Read the model definition and answer for the solid it produces. Units are mm, in the model's axes. Give positions to 0.01 mm unless a question says otherwise; leave off trailing zeros. Write each loop counter-clockwise with the first axis right and the second up, starting at its lowest first coordinate (ties: lowest second). Pieces come first, ordered by that corner, then holes. Notation, with made-up numbers: (39, 79.25) - (89, 79.25) arc R8 cw to (89, 91.25) - close; hole circle Ø3 at (28.25, 58.5). An arc over 180 degrees is marked (long way). Answer as CSV lines item,"result".
Autodesk Fusion 360 part; units mm, degrees
sketch "Sketch1" plane through (0, 0, 0) normal (0, 0, 1) x (1, 0, 0)
  line L0 (-100, 50) -> (300, 50)
  line L1 (300, 50) -> (300, -350)
  line L2 (300, -350) -> (-100, -350)
  line L3 (-100, -350) -> (-100, 50)
  dimension "d1" = 400
  dimension "d2" = 400
extrude "Extrude1" add sketch "Sketch1" along normal blind 3
sketch "Sketch2" plane through (0, 0, 3) normal (0, 0, 1) x (-1, 0, 0)
  line L0 (100, 350) -> (-300, 350)
  line L1 (-300, 350) -> (-300, -50)
  line L2 (-300, -50) -> (100, -50)
  line L3 (100, -50) -> (100, 350)
  line L4 (-263.3486, -40) -> (-290, -13.1239)
  line L5 (-290, -13.1239) -> (-270.7994, 7.2868)
  line L6 (-270.7994, 7.2868) -> (-243.7577, -19.9951)
  line L7 (-243.7577, -19.9951) -> (-263.3486, -40)
  circle A0 centre (-263.3392, -37.3821) radius 1
  circle A1 centre (-287.4151, -13.0924) radius 1
  circle A2 centre (-246.3371, -20.0207) radius 1
  circle A3 centre (-270.413, 4.269) radius 1
  line L8 (-105, 220) -> (-270, 220)
  line L9 (-270, 220) -> (-270, 320)
  line L10 (-270, 320) -> (-105, 320)
  line L11 (-105, 320) -> (-105, 220)
  circle A4 centre (-130.5, 232.5) radius 2.5
  circle A5 centre (-130.5, 307.5) radius 2.5
  circle A6 centre (-182.5, 232.5) radius 2.5
  circle A7 centre (-182.5, 307.5) radius 2.5
  line L12 (-152.9998, 228.0039) -> (-160.7739, 228.0044) construction
  line L13 (-160.7739, 228.0044) -> (-160.7741, 225.0005) construction
  line L14 (-160.7741, 225.0005) -> (-153, 225) construction
  line L15 (-153, 225) -> (-152.9998, 228.0039) construction
  line L16 (-153, 315) -> (-168.7144, 314.9704) construction
  line L17 (-168.7144, 314.9704) -> (-168.6983, 306.4348) construction
  line L18 (-168.6983, 306.4348) -> (-152.9839, 306.4644) construction
  line L19 (-152.9839, 306.4644) -> (-153, 315) construction
  line L20 (-49.76, 127.68) -> (70, 127.68)
  circle A8 centre (67.5, 66.3) radius 1.25
  line L21 (70, 127.68) -> (70, 63.8)
  circle A9 centre (-47.26, 125.18) radius 1.25
  circle A10 centre (67.5, 125.18) radius 1.25
  line L22 (-49.76, 63.8) -> (-49.76, 127.68)
  circle A11 centre (-47.26, 66.3) radius 1.25
  line L23 (70, 63.8) -> (-49.76, 63.8)
  line L24 (70, -20) -> (6.9, -20)
  line L25 (70, 33.8) -> (70, -20)
  line L26 (6.9, -20) -> (6.9, 33.8)
  circle A12 centre (9.4, 31.3) radius 1.25
  circle A13 centre (9.4, -17.5) radius 1.25
  circle A14 centre (67.5, 31.3) radius 1.25
  circle A15 centre (67.5, -17.5) radius 1.25
  line L27 (6.9, 33.8) -> (70, 33.8)
  circle A16 centre (67.5, 197.68) radius 1.25
  line L28 (70, 157.68) -> (28.7, 157.68)
  circle A17 centre (67.5, 160.18) radius 1.25
  line L29 (70, 200.18) -> (70, 157.68)
  circle A18 centre (31.2, 197.68) radius 1.25
  line L30 (28.7, 200.18) -> (70, 200.18)
  line L31 (28.7, 157.68) -> (28.7, 200.18)
  circle A19 centre (31.2, 160.18) radius 1.25
  dimension "d5" = 2
  dimension "d6" = 2
  dimension "d7" = 2
  dimension "d8" = 2
  dimension "d9" = 34.2
  dimension "d10" = 24.3
  dimension "d11" = 34.2
  dimension "d12" = 24.3
  dimension "d13" = 37.85
  dimension "d14" = 28
  dimension "d15" = 1.85
  dimension "d16" = 1.85
  dimension "d17" = 1.85
  dimension "d18" = 1.825
  dimension "d19" = 1.825
  dimension "d20" = 100
  dimension "d21" = 165
  dimension "d22" = 5
  dimension "d23" = 5
  dimension "d24" = 5
  dimension "d25" = 5
  dimension "d26" = 52
  dimension "d27" = 75
  dimension "d28" = 52
  dimension "d29" = 75
  dimension "d30" = 25.5
  dimension "d31" = 25.5
  dimension "d32" = 12.5
  dimension "d33" = 10
  dimension "d34" = 10
  dimension "d35" = 87.5
  dimension "d36" = 12.5
  dimension "d37" = 5
  dimension "d38" = 48
  dimension "d39" = 5
  dimension "d40" = 48
  dimension "d190" = 10
  dimension "d42" = 2.5
  dimension "d43" = 2.5
  dimension "d44" = 2.5
  dimension "d45" = 2.5
  dimension "d46" = 2.5
  dimension "d47" = 2.5
  dimension "d48" = 2.5
  dimension "d49" = 2.5
  dimension "d50" = 2.5
  dimension "d51" = 2.5
  dimension "d52" = 2.5
  dimension "d53" = 114.76
  dimension "d54" = 58.88
  dimension "d55" = 58.88
  dimension "d56" = 2.5
  dimension "d57" = 114.76
  dimension "d186" = 10
  dimension "d59" = 2.5
  dimension "d60" = 2.5
  dimension "d61" = 2.5
  dimension "d62" = 2.5
  dimension "d63" = 2.5
  dimension "d64" = 2.5
  dimension "d65" = 2.5
  dimension "d66" = 2.5
  dimension "d67" = 2.5
  dimension "d68" = 2.5
  dimension "d69" = 2.5
  dimension "d70" = 58.1
  dimension "d71" = 48.8
  dimension "d72" = 48.8
  dimension "d188" = 10
  dimension "d74" = 2.5
  dimension "d75" = 2.5
  dimension "d76" = 2.5
  dimension "d77" = 2.5
  dimension "d78" = 2.5
  dimension "d79" = 2.5
  dimension "d80" = 2.5
  dimension "d81" = 2.5
  dimension "d82" = 2.5
  dimension "d83" = 2.5
  dimension "d84" = 2.5
  dimension "d85" = 37.5
  dimension "d86" = 36.3
  dimension "d87" = 36.3
  dimension "d90" = 30
  dimension "d91" = 58.1
  dimension "d92" = 30
  dimension "d93" = 30
  dimension "d94" = 30
  dimension "d95" = 30
  dimension "d96" = 30
  dimension "d97" = 12.5
  dimension "d98" = 87.5
  dimension "d99" = 10
  dimension "d100" = 10
  dimension "d101" = 30
  dimension "d102" = 30
sketch "Sketch3" plane through (0, 0, 3) normal (0, 0, 1) x (1, 0, 0)
  line L0 (-100, -350.18) -> (75, -350.18)
  line L1 (75, -350.18) -> (75, -230.18)
  line L2 (75, -230.18) -> (-100, -230.18)
  line L3 (-100, -230.18) -> (-100, -350.18)
  line L4 (-28.7, -200.18) -> (-70, -200.18)
  line L5 (105, -320) -> (105, -220)
  dimension "d103" = 30
  dimension "d104" = 30
  dimension "d105" = 120
  dimension "d106" = 175
extrude "Extrude2" cut sketch "Sketch3" against normal blind 5.5
extrude "Extrude3" cut sketch "Sketch2" against normal blind 5.5 contours A4 | A5 | A6 | A7 | A8 | A9 | A10 | A11 | A12 | A13 | A14 | A15 | A16 | A17 | A18 | A19
extrude "Extrude4" cut sketch "Sketch2" against normal blind 5.5 contours A0 | A1 | A2 | A3
sketch "Sketch4" plane through (0, 0, 3) normal (0, 0, 1) x (-1, 0, 0)
  circle A0 centre (-270.413, 4.269) radius 1
  circle A1 centre (-287.4151, -13.0924) radius 1
  circle A2 centre (-246.3371, -20.0207) radius 1
  circle A3 centre (-263.3392, -37.3821) radius 1
  circle A4 centre (9.4, 31.3) radius 1.25
  circle A5 centre (-47.26, 125.18) radius 1.25
  circle A6 centre (31.2, 160.18) radius 1.25
  circle A7 centre (-130.5, 232.5) radius 2.5
  circle A8 centre (-182.5, 307.5) radius 2.5
  circle A9 centre (67.5, 197.68) radius 1.25
  circle A10 centre (-47.26, 66.3) radius 1.25
  circle A11 centre (9.4, -17.5) radius 1.25
  circle A12 centre (67.5, 31.3) radius 1.25
  circle A13 centre (67.5, 125.18) radius 1.25
  circle A14 centre (31.2, 197.68) radius 1.25
  circle A15 centre (-130.5, 307.5) radius 2.5
  circle A16 centre (-182.5, 232.5) radius 2.5
  circle A17 centre (67.5, 160.18) radius 1.25
  circle A18 centre (67.5, 66.3) radius 1.25
  circle A19 centre (67.5, -17.5) radius 1.25
  line L0 (-75, 230.18) -> (-75, 350)
  line L1 (-75, 350) -> (-300, 350)
  line L2 (-300, 350) -> (-300, -50)
  line L3 (-300, -50) -> (100, -50)
  line L4 (100, -50) -> (100, 230.18)
  line L5 (100, 230.18) -> (-75, 230.18)
  line L6 (-242.6879, 7.3358) -> (-100.7815, 7.3358)
  line L7 (-100.7815, 7.3358) -> (-100.7815, 199.5971)
  line L8 (-100.7815, 199.5971) -> (-242.6879, 199.5971)
  line L9 (-242.6879, 199.5971) -> (-242.6879, 7.3358)
  line L10 (-270.7994, 7.2868) -> (-243.7577, -19.9951)
  dimension "d113" = 20
  dimension "d114" = 40
extrude "Extrude5" cut sketch "Sketch4" against normal blind 3 contours L6 L7 L8 L9
sketch "Sketch5" plane through (0, 0, 3) normal (0, 0, 1) x (1, 0, 0)
  circle A0 centre (-90, 40) radius 1.5
  line L0 (-100, 50) -> (300, 50)
  line L1 (-100, -350) -> (-100, 50)
  circle A1 centre (290, 40) radius 1.5
  line L2 (300, 50) -> (300, -350)
  circle A2 centre (290, -340) radius 1.5
  line L3 (300, -350) -> (-100, -350)
  circle A3 centre (85, -340) radius 1.5
  line L4 (75, -230.18) -> (75, -350)
  circle A4 centre (-90, -220.18) radius 1.5
  line L5 (-100, -230.18) -> (75, -230.18)
  circle A5 centre (90.7815, 2.6642) radius 1.5
  line L6 (100.7815, -199.5971) -> (100.7815, -7.3358)
  line L7 (100.7815, -7.3358) -> (242.6879, -7.3358)
  circle A6 centre (252.6879, 2.6642) radius 1.5
  line L8 (242.6879, -7.3358) -> (242.6879, -199.5971)
  circle A7 centre (252.6879, -209.5971) radius 1.5
  line L9 (242.6879, -199.5971) -> (100.7815, -199.5971)
  circle A8 centre (85.7815, -214.5971) radius 1.5
  dimension "d117" = 3
  dimension "d118" = 10
  dimension "d119" = 10
  dimension "d120" = 3
  dimension "d121" = 10
  dimension "d122" = 10
  dimension "d123" = 3
  dimension "d124" = 10
  dimension "d125" = 10
  dimension "d126" = 3
  dimension "d127" = 10
  dimension "d128" = 10
  dimension "d129" = 3
  dimension "d130" = 10
  dimension "d131" = 10
  dimension "d132" = 3
  dimension "d133" = 10
  dimension "d134" = 10
  dimension "d135" = 3
  dimension "d136" = 10
  dimension "d137" = 10
  dimension "d138" = 3
  dimension "d139" = 10
  dimension "d140" = 10
  dimension "d141" = 3
  dimension "d142" = 15
  dimension "d143" = 15
extrude "Extrude6" cut sketch "Sketch5" against normal blind 3 contours A0 | A1 | A2 | A3 | A4 | A5 | A6 | A7 | A8
equation "d29 = d27"
(1) This flat-tipped pin is pushed along its axis until it touches: P1, Ø1.8, axis at x = 290, y = -340, coming from the -Z side. Where does it stop, or does it pass through?
Worked out:
P1,"passes through"
(2) A cutting plane is placed at A-A (x = 224). Write down the section's boundary in (y, z).
Worked out:
outline,"(-350, 0) - (-199.6, 0) - (-199.6, 3) - (-350, 3) - close; (-7.34, 0) - (50, 0) - (50, 3) - (-7.34, 3) - close"
(3) A cutting plane is placed at D-D (z = 2.5). Count the separate pieces of the cut face and the enclosed holes in it, and give its area (3 significant figures).
Worked out:
separate pieces,"1"
enclosed holes,"30"
area,"112,000 mm^2"
(4) A cutting plane is placed at C-C (y = -273). Write down the section's boundary in (x, z), and give its area (3 significant figures).
Worked out:
outline,"(75, 0) - (300, 0) - (300, 3) - (75, 3) - close"
area,"675 mm^2"
(5) A cutting plane is placed at B-B (y = -168.5). Write down the section's boundary in (x, z).
Worked out:
outline,"(-100, 0) - (100.78, 0) - (100.78, 3) - (-100, 3) - close; (242.69, 0) - (300, 0) - (300, 3) - (242.69, 3) - close"
(6) Find the intervals of material crossed by L1, parallel to Y at x = 47.26, z = 1.7; L2, parallel to Y at x = 182.5, z = 1.05; L3, parallel to X at y = -66.3, z = 1.55, in increasing order.
Worked out:
L1,"y = -230.18 to -126.43, -123.93 to -67.55, -65.05 to 50"
L2,"y = -350 to -310, -305 to -235, -230 to -199.6, -7.34 to 50"
L3,"x = -100 to -68.75, -66.25 to 46.01, 48.51 to 100.78, 242.69 to 300"
